For this review, use the dimensioned drawing (mm, ordinates from the lowest corner) and the shaded views. Coordinates: 2 decimals unless noted, no trailing zeros. Loops run counter-clockwise (first coordinate to the right, second up) from the corner with the lowest first, then second, coordinate; pieces in that order, holes last. Notation, with made-up numbers: M -4.75,29.25 L 21.25,29.25 A12 ccw 21.25,51.25 Z; hole C 84,9.25 d3. An arc over 180 degrees is marked long. Write item = value, one per line.
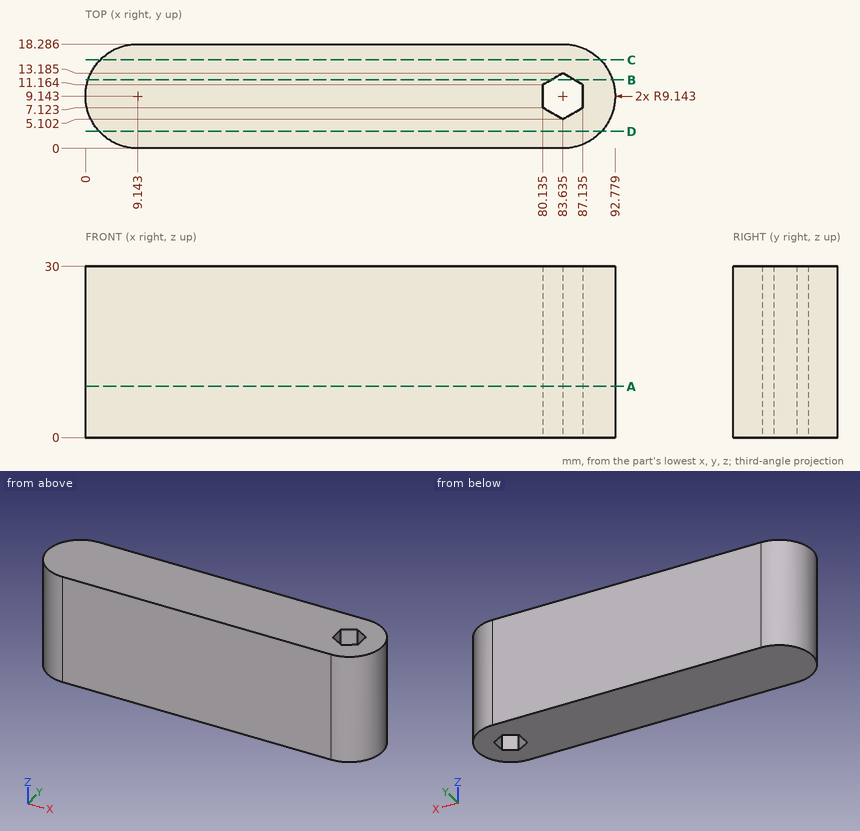
Q1. Add section C-C (y = 15.5). Write out the cut boundary in (x, z).
Solved:
outline = M 2.57,0 L 90.21,0 L 90.21,30 L 2.57,30 Z
Q2. For line 1 along X through (y, z) = (7.75, 16) (1 decimal); line 2 along X through (y, z) = (5.5, 6.5) (1 decimal); line 3 along X through (y, z) = (2.75, 17.25) (1 decimal), list the stretches that pass through material, from the lowest coordinate up.
Solved:
line_1 = 0.1 to 80.1, 87.1 to 92.7
line_2 = 0.8 to 82.9, 84.3 to 92
line_3 = 2.6 to 90.2
Q3. For pin 1 Ø4 at (y, z) = (7, 9.5) entering from +X; pin 2 Ø5 at (y, z) = (3, 9) entering from +X; pin 3 Ø5 at (y, z) = (12.5, 12.5) entering from +X, all flat-tipped, find the tip position at first contact; note any pin that passes through.
Solved:
pin_1 = 92.78
pin_2 = 92.02
pin_3 = 92.74
Q4. Add section A-A (z = 9). Write out the cut boundary in (x, y) (1 decimal), and give its area (3 significant figures).
Solved:
outline = M 9.1,0 L 83.6,0 A9.1 ccw 83.6,18.3 L 9.1,18.3 A9.1 ccw Z; hole M 80.1,7.1 L 83.6,5.1 L 87.1,7.1 L 87.1,11.2 L 83.6,13.2 L 80.1,11.2 Z
area = 1,580 mm²
Q5. Add section B-B (y = 12). Write out the cut boundary in (x, z).
Solved:
outline = M 0.46,0 L 81.58,0 L 81.58,30 L 0.46,30 Z; M 85.69,0 L 92.32,0 L 92.32,30 L 85.69,30 Z
Q6. Add section D-D (y = 3). Write out the cut boundary in (x, z).
Solved:
outline = M 2.37,0 L 90.41,0 L 90.41,30 L 2.37,30 Z
